from build123d import *

# Parameters (mm, degrees)
F3_DEPTH = 4


with BuildPart() as f1:
    # F0 (on Front) → F1 (revolve)
    with BuildSketch(Plane.XZ):
        Polygon((0, 3), (0, 0), (35, 0), (35, 4), (26, 4), (26, 7), (21, 7), (21, 3), align=None)
    revolve(axis=Axis((0, 0, 21.586414), (0, 0, 1)))

    # F2 (on face) → F3 (cut)
    with BuildSketch(Plane.XY.offset(4)):
        with BuildLine():
            ThreePointArc((2.75, 30), (-0.063037, 32.749277), (-2.74711, 29.873958))
            ThreePointArc((-2.74711, 29.873958), (0, 27.25), (2.74711, 29.873958))
            ThreePointArc((2.74711, 29.873958), (2.749277, 29.936963), (2.75, 30))
        make_face()
        with BuildLine():
            ThreePointArc((-27.25, 0), (-28.011393, 1.899459), (-29.873958, 2.74711))
            ThreePointArc((-29.873958, 2.74711), (-32.75, 0), (-29.873958, -2.74711))
            ThreePointArc((-29.873958, -2.74711), (-28.011393, -1.899459), (-27.25, 0))
        make_face()
        with BuildLine():
            ThreePointArc((2.74711, -29.873958), (0, -27.25), (-2.74711, -29.873958))
            ThreePointArc((-2.74711, -29.873958), (-0.063037, -32.749277), (2.75, -30))
            ThreePointArc((2.75, -30), (2.749277, -29.936963), (2.74711, -29.873958))
        make_face()
        with BuildLine():
            ThreePointArc((32.75, 0), (31.899459, 1.988607), (29.873958, 2.74711))
            ThreePointArc((29.873958, 2.74711), (27.25, 0), (29.873958, -2.74711))
            ThreePointArc((29.873958, -2.74711), (31.899459, -1.988607), (32.75, 0))
        make_face()
    extrude(amount=-F3_DEPTH, mode=Mode.SUBTRACT)


solid = f1.part
Design review of the part built by this model. Coordinates are the model's own, in mm. Coordinates: 2 decimals unless noted, no trailing zeros. Loops run counter-clockwise (first coordinate to the right, second up) from the corner with the lowest first, then second, coordinate; pieces in that order, holes last.
Item 1: Wall thickness on L1, parallel to Y at x = 0, z = 4.4; L2, parallel to Z at x = 18.5, y = 26; L3, parallel to Z at x = -13.5, y = 13.5: over which ranges is each line inside the solid? List them lowest first.
Completed:
L1: y = -26 to -21, 21 to 26
L2: z = 0 to 4
L3: z = 0 to 3
Item 2: Add section B-B (z = 1). Write out the cut boundary in (x, y).
Completed:
outline: circle Ø70 at (0, 0); hole (-29.87, -2.75) arc R2.75 ccw to (-27.25, 0) arc R2.75 ccw to (-29.87, 2.75) arc R2.75 ccw (long way) to start; hole (2.75, -30) arc R2.75 ccw to (2.75, -29.87) arc R2.75 ccw (long way) to start; hole (2.75, 29.87) arc R2.75 ccw to (2.75, 30) arc R2.75 ccw (long way) to start; hole (29.87, 2.75) arc R2.75 ccw (long way) to (32.75, 0) arc R2.75 ccw to start
Item 3: Draft analysis for pull direction Y (two halves, no side actions). For faces 1 (the flat face through (5, -26, 4)), 2 (the cylindrical face through (-20.633, -15.821, 5.521)), 3 (the cylindrical face through (20.03, 6.31, 4.97)), 4 (the flat face through (0, 0, 3)), state which applies: pulls with the +Y half, pulls with the -Y half, needs draft (parallel to the pull), parting line crosses it, or undercut.
Completed:
face 1: needs draft
face 2: parting line crosses it
face 3: undercut
face 4: undercut
Item 4: Add section A-A (x = 0). Write out the cut boundary in (y, z), and give its area (3 significant figures).
Completed:
outline: (-35, 0) - (-32.75, 0) - (-32.75, 4) - (-35, 4) - close; (-27.25, 0) - (27.25, 0) - (27.25, 4) - (26, 4) - (26, 7) - (21, 7) - (21, 3) - (-21, 3) - (-21, 7) - (-26, 7) - (-26, 4) - (-27.25, 4) - close; (32.75, 0) - (35, 0) - (35, 4) - (32.75, 4) - close
area: 224 mm2
Item 5: Add section C-C (y = -28.5). Write out the cut boundary in (x, z), and give its area (3 significant figures).
Completed:
outline: (-20.32, 0) - (-2.3, 0) - (-2.3, 4) - (-20.32, 4) - close; (2.3, 0) - (20.32, 0) - (20.32, 4) - (2.3, 4) - close
area: 144 mm2
Item 6: Clearance check with flat-ended pins moving along their axes: pin 1 (3 mm diameter, centred on x = -13, y = 22.5, fed in from -Z); pin 2 (2 mm diameter, centred on x = 6.5, z = 2, fed in from -Y); pin 3 (3 mm diameter, centred on x = -11.5, z = 2.5, fed in from -Y); pin 4 (1 mm diameter, centred on y = 24.5, z = 6, fed in from +X). State where each tip first meets the part, or that it passes through.
Completed:
pin 1: stops at z = 0
pin 2: stops at y = -34.57
pin 3: stops at y = -33.54
pin 4: stops at x = 10
Item 7: Add section D-D (z = 5.75). Write out the cut boundary in (x, y), and give its area (3 significant figures).
Completed:
outline: circle Ø52 at (0, 0); hole circle Ø42 at (0, 0)
area: 738 mm2
